```python
from build123d import *

# Parameters (mm, degrees)
SKETCH_1_R               = 148.209
SKETCH_1_R_2             = 144.78
EXTRUDE_1_DEPTH          = 500
SKETCH_2_W               = 10
SKETCH_2_H               = 30
PATTERN_CIRCULAR_1_COUNT = 4


with BuildPart() as part:
    # 草圖1 → 填料-伸長1 (new body)
    with BuildSketch(Plane.XY):
        Circle(SKETCH_1_R)
        Circle(SKETCH_1_R_2, mode=Mode.SUBTRACT)
    extrude(amount=EXTRUDE_1_DEPTH)

    # 草圖2 → 除料-旋轉1 (revolve, cut)
    with BuildSketch(Plane(origin=(0, 0, 0), x_dir=(0, 0, -1), z_dir=(1, 0, 0))):
        with Locations((-405, 148.209)):
            Rectangle(SKETCH_2_W, SKETCH_2_H)
    cut_revolve_1 = revolve(axis=Axis((0, 133.209, 400), (0, 1, 0)), mode=Mode.SUBTRACT)

    # 環狀複製排列1: 除料-旋轉1 ×4 about axis
    pattern_circular_1_axis = Axis((0, 0, 500), (0, 0, -1))
    for i in range(1, PATTERN_CIRCULAR_1_COUNT):
        add(cut_revolve_1.rotate(pattern_circular_1_axis, i * 360 / PATTERN_CIRCULAR_1_COUNT), mode=Mode.SUBTRACT)


solid = part.part
```
Part model, mm, in its own coordinate system. Round coordinates to 2 decimals unless told otherwise and drop trailing zeros. Write each loop counter-clockwise with the first axis right and the second up, starting at its lowest first coordinate (ties: lowest second). Pieces come first, ordered by that corner, then holes. Notation, with made-up numbers: (-15.75, 0) -> (-1.75, 0) arc R29 cw to (-1.75, 25) -> close; hole circle Ø8 at (-12.75, 58). An arc over 180 degrees is marked (long way). Return JSON: item names as keys, results as strings. Group by question number.
Q1. Saw through at A-A on y = 0. Write the cut outline in (x, z).
Q2. Mould opens along X. For faces 1 (the flat face through (32, -142, 500)), 2 (the cylindrical face through (-32.129, -144.685, 246.5)), 3 (the cylindrical face through (0, -146, 390)) say: pulls with the +X half, pulls with the -X half, needs draft (parallel to the pull), parting line crosses it, or undercut.
Q3. Pin check, flat tips, straight feed: pin 1 (1.5 mm diameter, centred on x = -8, z = 239.5, fed in from +Y); pin 2 (1.5 mm diameter, centred on y = 66, z = 309, fed in from +X); pin 3 (1 mm diameter, centred on x = 107.5, z = 174.5, fed in from -Y); pin 4 (18 mm diameter, centred on x = 0, z = 400, fed in from -Y). Stop position of each tip, or through.
Q4. Probe L1, parallel to X at y = 0, z = 314; L2, parallel to Z at x = 0, y = 145; L3, parallel to Y at x = 111, z = 132. List the from-to ranges inside material, lowest first. Write a range as [from, to].
Q5. Saw through at D-D on y = 125.5. Write the cut outline in (x, z).
Answer:
{
 "1": {"outline": "(-148.21, 0) -> (-144.78, 0) -> (-144.78, 390) -> (-148.21, 390) -> close; (-148.21, 410) -> (-144.78, 410) -> (-144.78, 500) -> (-148.21, 500) -> close; (144.78, 0) -> (148.21, 0) -> (148.21, 390) -> (144.78, 390) -> close; (144.78, 410) -> (148.21, 410) -> (148.21, 500) -> (144.78, 500) -> close"},
 "2": {"face 1": "needs draft", "face 2": "parting line crosses it", "face 3": "undercut"},
 "3": {"pin 1": "y = 148.03", "pin 2": "x = 133.07", "pin 3": "y = -102.55", "pin 4": "through"},
 "4": {"L1": "[-148.21, -144.78], [144.78, 148.21]", "L2": "[0, 390], [410, 500]", "L3": "[-98.21, -92.95], [92.95, 98.21]"},
 "5": {"outline": "(-78.84, 0) -> (-72.19, 0) -> (-72.19, 500) -> (-78.84, 500) -> close; (72.19, 0) -> (78.84, 0) -> (78.84, 500) -> (72.19, 500) -> close"}
}
